from build123d import *

# Parameters (mm, degrees)
F2_R     = 9.5
F3_R     = 6
F4_R     = 45.15
F4_R_2   = 42.15
F5_DEPTH = 1
F4_R_3   = 24.2
F4_R_4   = 23.2
F6_DEPTH = 0.5


with BuildPart() as f1:
    # F0 (on Front) → F1 (revolve)
    with BuildSketch(Plane.XZ):
        Polygon((53.5, 22.2), (23.2, 22.2), (23.2, 18.5), (45.15, 18.5), (45.15, 0), (53.5, 0), align=None)
    revolve(axis=Axis((0, 0, 3.413312), (0, 0, -1)))

    # F2
    f2_edges = [f1.edges().sort_by_distance(p)[0] for p in [
        (-53.5, 0, 22.2),
    ]]
    fillet(f2_edges, radius=F2_R)

    # F3
    f3_edges = [f1.edges().sort_by_distance(p)[0] for p in [
        (-53.5, 0, 0),
    ]]
    fillet(f3_edges, radius=F3_R)

    # F4 (on face) → F5 (cut)
    with BuildSketch(Plane(origin=(0, 0, 18.5), x_dir=(1, 0, 0), z_dir=(0, 0, -1))):
        Circle(F4_R)
        Circle(F4_R_2, mode=Mode.SUBTRACT)
    extrude(amount=-F5_DEPTH, mode=Mode.SUBTRACT)

    # F4 (on face) → F6 (cut)
    with BuildSketch(Plane(origin=(0, 0, 18.5), x_dir=(1, 0, 0), z_dir=(0, 0, -1))):
        Circle(F4_R_3)
        Circle(F4_R_4, mode=Mode.SUBTRACT)
    extrude(amount=-F6_DEPTH, mode=Mode.SUBTRACT)


solid = f1.part
Can you work these out from the model? Positions are in its coordinate system, mm. A direction names the side the tool comes from. Coordinates: 2 decimals unless noted, no trailing zeros. Write each loop counter-clockwise with the first axis right and the second up, starting at its lowest first coordinate (ties: lowest second). Pieces come first, ordered by that corner, then holes. Notation, with made-up numbers: (87, -12.5) -> (146, -12.5) arc R17 cw to (146, -8.5) -> close; hole circle Ø7 at (-17.5, -28.75). An arc over 180 degrees is marked (long way). Write item = value, one per line.
(1) Imagine slicing it at C-C (z = 7.75). Please give me the cut outline in (x, y).
Verdict:
outline = circle Ø107 at (0, 0); hole circle Ø90.3 at (0, 0)
(2) Imagine slicing it at D-D (z = 2.25). Please give me the cut outline in (x, y), and give its area (3 significant figures).
Verdict:
outline = circle Ø104.37 at (0, 0); hole circle Ø90.3 at (0, 0)
area = 2,150 mm^2
(3) For pin 1 (1 mm diameter, centred on x = 27, y = -26.5, fed in from -Z); pin 2 (12 mm diameter, centred on y = -12.5, z = 3, fed in from -X); pin 3 (2 mm diameter, centred on x = -41, z = 8.5, fed in from -Y), each with a flat end and sliding along its axis, tell me the tip position at first contact or that it passes through.
Verdict:
pin_1 = 18.5
pin_2 = -53.01
pin_3 = -35.53
(4) On a 3-axis mill with a long thin cutter (end or side, diameter ignored), from which of +Z, -Z, +X, -X, +Y, -Y can I reach the whole of each face in a straight line? I mean faces 4 (the face through (-14, 40, 19.5)), 5 (the face through (19, 19, 22.2)). Say none if no direction works.
Verdict:
face_4 = -Z
face_5 = +Z, +X, -X, +Y, -Y
(5) Imagine slicing it at A-A (y = 0). Please give me the cut outline in (x, z), and give its area (3 significant figures).
Verdict:
outline = (-53.5, 6) arc R6 ccw to (-47.5, 0) -> (-45.15, 0) -> (-45.15, 19.5) -> (-42.15, 19.5) -> (-42.15, 18.5) -> (-24.2, 18.5) -> (-24.2, 19) -> (-23.2, 19) -> (-23.2, 22.2) -> (-44, 22.2) arc R9.5 ccw to (-53.5, 12.7) -> close; (23.2, 19) -> (24.2, 19) -> (24.2, 18.5) -> (42.15, 18.5) -> (42.15, 19.5) -> (45.15, 19.5) -> (45.15, 0) -> (47.5, 0) arc R6 ccw to (53.5, 6) -> (53.5, 12.7) arc R9.5 ccw to (44, 22.2) -> (23.2, 22.2) -> close
area = 472 mm^2
(6) If I drill on probe 1 along X at (y, z) = (0, 18.7); probe 2 along Y at (x, z) = (0, 11); probe 3 along X at (y, z) = (0, 13.25), over which ranges is the centre line in solid material (lowest first)?
Verdict:
probe_1 = -51.37 to -45.15, -42.15 to -24.2, 24.2 to 42.15, 45.15 to 51.37
probe_2 = -53.5 to -45.15, 45.15 to 53.5
probe_3 = -53.48 to -45.15, 45.15 to 53.48
(7) Thinking about a two-plate mould opening in X: for faces 1 (the face through (-42, 17, 0)), 2 (the face through (-11.598, 52.228, 9.397)), 3 (the face through (-23.178, -1.02, 20.578)), which applies, +X half, -X half, draft (parallel to the pull), parting line (faces both ways), or undercut?
Verdict:
face_1 = draft
face_2 = parting line
face_3 = undercut
